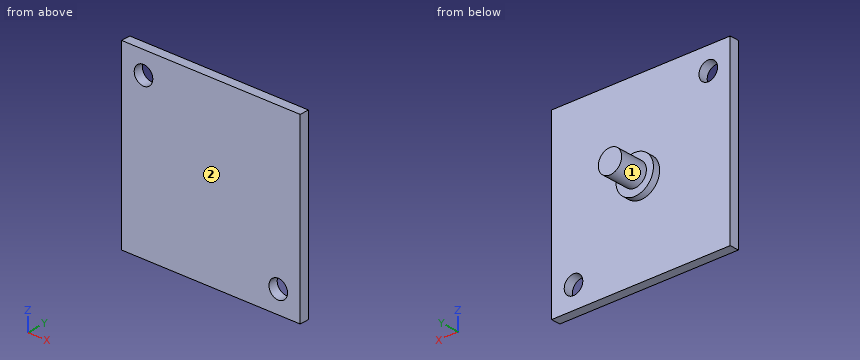
```python
from build123d import *

# Parameters (mm, degrees)
SKETCH1_W           = 38.1
SKETCH1_H           = 38.1
SKETCH1_R           = 1.984375
BOSS_EXTRUDE1_DEPTH = 2
SKETCH2_R           = 4.0005
BOSS_EXTRUDE2_DEPTH = 1.508000032
SKETCH3_R           = 2.5
BOSS_EXTRUDE3_DEPTH = 6


with BuildPart() as part:
    # Sketch1 → Boss-Extrude1 (new body)
    with BuildSketch(Plane(origin=(0, 0, 0), x_dir=(1, 0, 0), z_dir=(0, 1, 0))):
        Rectangle(SKETCH1_W, SKETCH1_H)
        with Locations(Location((14.368409794, 14.368409794, 0), (0, 0, 270))):
            Circle(SKETCH1_R, mode=Mode.SUBTRACT)
        with Locations(Location((-14.368409794, -14.368409794, 0), (0, 0, 90))):
            Circle(SKETCH1_R, mode=Mode.SUBTRACT)
    extrude(amount=BOSS_EXTRUDE1_DEPTH)

    # Sketch2 → Boss-Extrude2 (add)
    with BuildSketch(Plane(origin=(0, 2, 0), x_dir=(1, 0, 0), z_dir=(0, 1, 0))):
        with Locations(Location((0, 0, 0), (0, 0, 90))):
            Circle(SKETCH2_R)
    extrude(amount=BOSS_EXTRUDE2_DEPTH)

    # Sketch3 → Boss-Extrude3 (add)
    with BuildSketch(Plane(origin=(0, 3.508000032, 0), x_dir=(1, 0, 0), z_dir=(0, 1, 0))):
        with Locations(Location((0, 0, 0), (0, 0, 270))):
            Circle(SKETCH3_R)
    extrude(amount=BOSS_EXTRUDE3_DEPTH)


solid = part.part
```
Geometry: final body of the model. Coordinates: model frame, mm. Face numbers are marked on the shaded views. A direction names the side the tool comes from. Give positions to 0.01 mm unless a question says otherwise; leave off trailing zeros. Loops run counter-clockwise (first coordinate to the right, second up) from the corner with the lowest first, then second, coordinate; pieces in that order, holes last. Notation, with made-up numbers: (63, 58.5) -> (118, 58.5) arc R14 cw to (118, 76.5) -> close; hole circle Ø4 at (-13.5, 31.5). An arc over 180 degrees is marked (long way). Use CSV: the item, a comma, the result in double quotes.
(1) Cut plane B-B (z = -13). Output: boundary loops of the cut face in (x, y).
From the geometry:
outline,"(-19.05, 0) -> (12.93, 0) -> (12.93, 2) -> (-19.05, 2) -> close; (15.81, 0) -> (19.05, 0) -> (19.05, 2) -> (15.81, 2) -> close"
(2) Access query for the marked faces 1 and 2. Directions: +Z, -Z, +X, -X, +Y, -Y. A direction counts if a zero-diameter tool reaches every point of the face in a straight line with its end or side. Return the directions, or none.
From the geometry:
face 1,"+Y"
face 2,"+Z, -Z, +X, -X, -Y"
(3) Cut plane D-D (z = 0). Output: boundary loops of the cut face in (x, y), plus the area to 3 significant figures.
From the geometry:
outline,"(-19.05, 0) -> (19.05, 0) -> (19.05, 2) -> (4, 2) -> (4, 3.51) -> (2.5, 3.51) -> (2.5, 9.51) -> (-2.5, 9.51) -> (-2.5, 3.51) -> (-4, 3.51) -> (-4, 2) -> (-19.05, 2) -> close"
area,"118 mm^2"
(4) Cut plane C-C (x = -13.5). Output: boundary loops of the cut face in (y, z).
From the geometry:
outline,"(0, -19.05) -> (2, -19.05) -> (2, 12.58) -> (0, 12.58) -> close; (0, 16.15) -> (2, 16.15) -> (2, 19.05) -> (0, 19.05) -> close"
(5) First-contact query: P1, Ø11.5, axis at x = 5.5, z = -1, coming from the +Y side; P2, Ø1.5, axis at y = 7, z = -2, coming from the +X side; P3, Ø1.5, axis at x = -10.5, z = 3.5, coming from the +Y side. Flat tips, straight axial feed; report the tip coordinate or a pass-through.
From the geometry:
P1,"y = 9.51"
P2,"x = 2.17"
P3,"y = 2"
(6) Cut plane A-A (x = 0). Output: boundary loops of the cut face in (y, z).
From the geometry:
outline,"(0, -19.05) -> (2, -19.05) -> (2, -4) -> (3.51, -4) -> (3.51, -2.5) -> (9.51, -2.5) -> (9.51, 2.5) -> (3.51, 2.5) -> (3.51, 4) -> (2, 4) -> (2, 19.05) -> (0, 19.05) -> close"
(7) Ray query, line 1 along Y through (x, z) = (-4, 2.5); line 2 along X through (y, z) = (5, 2); line 3 along X through (y, z) = (9.25, -1). Return the intervals inside material, ascending. Write a range as [from, to].
From the geometry:
line 1,"[0, 2]"
line 2,"[-1.5, 1.5]"
line 3,"[-2.29, 2.29]"
